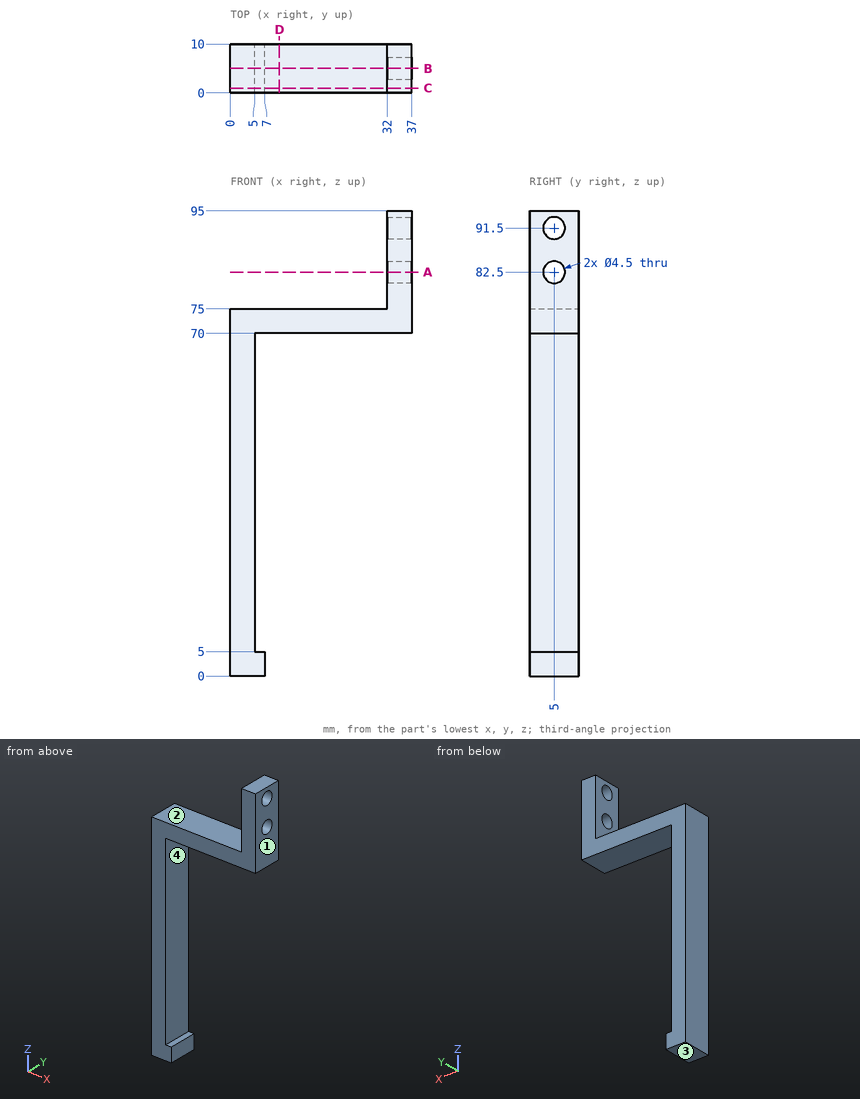
Could you check a few things on this drawing? It's one solid part, dimensions in mm from its lowest x, y, z. Coordinates: 2 decimals unless noted, no trailing zeros. Write each loop counter-clockwise with the first axis right and the second up, starting at its lowest first coordinate (ties: lowest second). Pieces come first, ordered by that corner, then holes. Notation, with made-up numbers: (-17.5, 0) - (21.5, 0) arc R18 ccw to (21.5, 13) - close; hole circle Ø2 at (32, -27.75). An arc over 180 degrees is marked (long way). Put each result on its own line as item: value. Start each with the question number.
Q1. Please list where these lines run through material, in increasing order: L1, parallel to Y at x = 33, z = 82.5; L2, parallel to Z at x = 6.5, y = 3.5; L3, parallel to X at y = 9, z = 85.
Q2. I want a section at C-C on y = 1. Write out the boundary of the cut face in (x, z).
Q3. I want a section at D-D on x = 10. Write out the boundary of the cut face in (y, z), plus the area to 3 significant figures.
Q4. Thinking about a two-plate mould opening in Z: for the marked faces 1, 2, 3 and 4, which applies, pulls with the +Z half, pulls with the -Z half, needs draft (parallel to the pull), parting line crosses it, or undercut?
Q5. I want a section at A-A on z = 82.5. Write out the boundary of the cut face in (x, y).
Q6. I want a section at B-B on y = 5. Write out the boundary of the cut face in (x, z), plus the area to 3 significant figures.
Q7. I'm going to push flat-ended pins straight in: P1, Ø6, axis at x = 25, y = 8.5, coming from the +Z side; P2, Ø4, axis at y = 8, z = 67.5, coming from the +X side; P3, Ø1.5, axis at y = 5, z = 2.5, coming from the +X side. Where does each tip first touch, or does it pass through?
Checks:
1. L1: 0 to 2.75, 7.25 to 10
1. L2: 0 to 5, 70 to 75
1. L3: 32 to 37
2. outline: (0, 0) - (7, 0) - (7, 5) - (5, 5) - (5, 70) - (37, 70) - (37, 95) - (32, 95) - (32, 75) - (0, 75) - close
3. outline: (0, 70) - (10, 70) - (10, 75) - (0, 75) - close
3. area: 50.0 mm²
4. face 1: needs draft
4. face 2: pulls with the +Z half
4. face 3: pulls with the -Z half
4. face 4: undercut
5. outline: (32, 0) - (37, 0) - (37, 2.75) - (32, 2.75) - close; (32, 7.25) - (37, 7.25) - (37, 10) - (32, 10) - close
6. outline: (0, 0) - (7, 0) - (7, 5) - (5, 5) - (5, 70) - (37, 70) - (37, 80.25) - (32, 80.25) - (32, 75) - (0, 75) - close; (32, 84.75) - (37, 84.75) - (37, 89.25) - (32, 89.25) - close; (32, 93.75) - (37, 93.75) - (37, 95) - (32, 95) - close
6. area: 600 mm²
7. P1: z = 75
7. P2: x = 5
7. P3: x = 7
